from build123d import *

# Parameters (mm, degrees)
F1_DEPTH = 406.4
F2_SIZE  = 19.04999
F3_SIZE  = 19.04999


# Not quite as in the source:
# - a fillet or chamfer is up to 0.001 mm smaller than in the source, because OpenCascade refuses the exact size


with BuildPart() as f1:
    # F0 (on Front) → F1 (new body)
    with BuildSketch(Plane.XZ):
        Polygon((333.375, 9.525), (-333.375, 9.525), (-314.325, -9.525), (314.325, -9.525), align=None)
    extrude(amount=-F1_DEPTH)

    # F2 (size 19.05 in the source; OpenCascade refuses exactly that, so slightly less here)
    f2_edges = [f1.edges().sort_by_distance(p)[0] for p in [
        (0, 406.4, -9.525),
    ]]
    chamfer(f2_edges, length=F2_SIZE)

    # F3 (size 19.05 in the source; OpenCascade refuses exactly that, so slightly less here)
    f3_edges = [f1.edges().sort_by_distance(p)[0] for p in [
        (0, 0, -9.525),
    ]]
    chamfer(f3_edges, length=F3_SIZE)


solid = f1.part
Geometry: final body of the model. Coordinates: model frame, mm. Give positions to 0.01 mm unless a question says otherwise; leave off trailing zeros. Loops run counter-clockwise (first coordinate to the right, second up) from the corner with the lowest first, then second, coordinate; pieces in that order, holes last. Notation, with made-up numbers: (-7, 59) - (24, 59) arc R15 cw to (24, 74) - close; hole circle Ø7 at (30, 28.25). An arc over 180 degrees is marked (long way). Answer as CSV lines item,"result". Start each with the question number.
1. Pin query (flat end, axial travel): P1, Ø4, axis at x = 251.5, z = 4.5, coming from the -Y side (3 decimals); P2, Ø1.5, axis at x = -226, z = 0, coming from the +Y side (3 decimals); P3, Ø1, axis at x = -83.5, z = 3.5, coming from the -Y side (3 decimals). Return the tip coordinate at first contact, or that it passes through.
2. Section C-C, the plane z = 1.75. Return loops of the section in (x, y) (3 decimals), plus the area to 3 significant figures.
3. Section B-B, the plane y = 370.5. Return loops of the section in (x, z) (3 decimals).
4. Ray query, L1, parallel to X at y = 218, z = -6.75; L2, parallel to X at y = 47, z = 4.5; L3, parallel to Y at x = 147, z = -8.5 (3 decimals). Return the intervals inside material, ascending.
Answers:
1,P1,"stops at y = 3.025"
1,P2,"stops at y = 397.625"
1,P3,"stops at y = 5.525"
2,outline,"(-325.6, 7.775) - (325.6, 7.775) - (325.6, 398.625) - (-325.6, 398.625) - close"
2,area,"255,000 mm2"
3,outline,"(-333.375, 9.525) - (-314.325, -9.525) - (314.325, -9.525) - (333.375, 9.525) - close"
4,L1,"x = -317.1 to 317.1"
4,L2,"x = -328.35 to 328.35"
4,L3,"y = 18.025 to 388.375"
